from build123d import *

# Parameters (mm, degrees)
SKETCH1_R           = 76.2
SKETCH1_R_2         = 2.54
BOSS_EXTRUDE1_DEPTH = 19.05
SKETCH2_W           = 3.175
SKETCH2_H           = 6.35


with BuildPart() as part:
    # Sketch1 → Boss-Extrude1 (new body)
    with BuildSketch(Plane(origin=(0, 0, 0), x_dir=(1, 0, 0), z_dir=(0, 1, 0))):
        Circle(SKETCH1_R)
        Circle(SKETCH1_R_2, mode=Mode.SUBTRACT)
        with Locations((25.4, -25.4)):
            Circle(SKETCH1_R_2, mode=Mode.SUBTRACT)
        with Locations((50.8, -25.4)):
            Circle(SKETCH1_R_2, mode=Mode.SUBTRACT)
    extrude(amount=BOSS_EXTRUDE1_DEPTH)

    # Sketch2 → Cut-Revolve1 (revolve, cut)
    with BuildSketch(Plane.XY):
        with Locations((-74.6125, 9.525)):
            Rectangle(SKETCH2_W, SKETCH2_H)
    revolve(axis=Axis((0, 4.7625, 0), (0, 1, 0)), mode=Mode.SUBTRACT)


solid = part.part
Input: part model. Units: mm. Frame: model coordinates. A direction names the side the tool comes from. Round coordinates to 2 decimals unless told otherwise and drop trailing zeros. Loops run counter-clockwise (first coordinate to the right, second up) from the corner with the lowest first, then second, coordinate; pieces in that order, holes last. Notation, with made-up numbers: M -3.75,58.25 L 8.25,58.25 A23 cw 8.25,91.25 Z; hole C -24,-34.75 d7. An arc over 180 degrees is marked long. Answer as CSV lines item,"result". Start each with the question number.
(1) Section D-D, the plane z = 25.4. Output: boundary loops of the cut face in (x, y).
(2) Section C-C, the plane x = 30.5. Output: boundary loops of the cut face in (y, z).
(3) Line query: line 1 (X direction, y = 13, z = 0); line 2 (X direction, y = 12.5, z = 25.4); line 3 (X direction, y = 13.5, z = 25.4). Output: solid intervals per line, ascending. Write a range as [from, to].
(4) Section B-B, the plane z = 0. Output: boundary loops of the cut face in (x, y) (3 decimals).
(5) Draft query along Z for faces 1 (the cylindrical face through (27.746, 9.392, 26.373)), 2 (the cylindrical face through (-60.47, 3.131, 46.367)), 3 (the flat face through (16, 19.05, -1)). Return one class per face: released by +Z, released by -Z, zero draft, split by the parting line, or undercut.
(6) First-contact query: pin 1 (6 mm diameter, centred on x = 25.4, z = 25.4, fed in from -Y); pin 2 (6 mm diameter, centred on x = -22.5, y = 13, fed in from -Z); pin 3 (3 mm diameter, centred on x = 49.5, y = 9, fed in from -Z); pin 4 (2 mm diameter, centred on y = 8.5, z = 29.5, fed in from -X). Flat tips, straight axial feed; report the tip coordinate or a pass-through.
(7) Section A-A, the plane x = 0. Output: boundary loops of the cut face in (y, z) (3 decimals).
(8) Reachability of faces 4 (the flat face through (16, 0, -1)), 5 (the cylindrical face through (9.506, 9.569, 72.404)) from +Z, -Z, +X, -X, +Y, -Y: full face, straight path, thin tool, end or side. Return the list, or none.
Values found:
1,outline,"M -71.84,0 L 22.86,0 L 22.86,19.05 L -71.84,19.05 L -71.84,12.7 L -68.47,12.7 L -68.47,6.35 L -71.84,6.35 Z; M 27.94,0 L 48.26,0 L 48.26,19.05 L 27.94,19.05 Z; M 53.34,0 L 71.84,0 L 71.84,6.35 L 68.47,6.35 L 68.47,12.7 L 71.84,12.7 L 71.84,19.05 L 53.34,19.05 Z"
2,outline,"M 0,-69.83 L 6.35,-69.83 L 6.35,-66.35 L 12.7,-66.35 L 12.7,-69.83 L 19.05,-69.83 L 19.05,69.83 L 12.7,69.83 L 12.7,66.35 L 6.35,66.35 L 6.35,69.83 L 0,69.83 Z"
3,line 1,"x = [-76.2, -2.54], [2.54, 76.2]"
3,line 2,"x = [-68.47, 22.86], [27.94, 48.26], [53.34, 68.47]"
3,line 3,"x = [-71.84, 22.86], [27.94, 48.26], [53.34, 71.84]"
4,outline,"M -76.2,0 L -2.54,0 L -2.54,19.05 L -76.2,19.05 L -76.2,12.7 L -73.025,12.7 L -73.025,6.35 L -76.2,6.35 Z; M 2.54,0 L 76.2,0 L 76.2,6.35 L 73.025,6.35 L 73.025,12.7 L 76.2,12.7 L 76.2,19.05 L 2.54,19.05 Z"
5,face 1,"undercut"
5,face 2,"split by the parting line"
5,face 3,"zero draft"
6,pin 1,"stops at y = 0"
6,pin 2,"stops at z = -73.66"
6,pin 3,"stops at z = -55.03"
6,pin 4,"stops at x = -67.23"
7,outline,"M 0,-76.2 L 6.35,-76.2 L 6.35,-73.025 L 12.7,-73.025 L 12.7,-76.2 L 19.05,-76.2 L 19.05,-2.54 L 0,-2.54 Z; M 0,2.54 L 19.05,2.54 L 19.05,76.2 L 12.7,76.2 L 12.7,73.025 L 6.35,73.025 L 6.35,76.2 L 0,76.2 Z"
8,face 4,"+Z, -Z, +X, -X, -Y"
8,face 5,"none"
